Read the model definition and answer for the solid it produces. Units are mm, in the model's axes. A direction names the side the tool comes from. Coordinates: 2 decimals unless noted, no trailing zeros. Loops run counter-clockwise (first coordinate to the right, second up) from the corner with the lowest first, then second, coordinate; pieces in that order, holes last. Notation, with made-up numbers: (-23.5, -30) -> (29.5, -30) arc R24 ccw to (29.5, -2) -> close; hole circle Ø2 at (-25.75, 7). An arc over 180 degrees is marked (long way). Answer as CSV lines item,"result".
```python
from build123d import *

# Parameters (mm, degrees)
CROQUIS1_W                 = 19.8
CROQUIS1_H                 = 11.5
SALIENTE_EXTRUIR1_DEPTH    = 70.5
VACIADO1_T                 = -2
CROQUIS4_W                 = 15.8
CROQUIS4_H                 = 28
CORTAR_EXTRUIR1_DEPTH      = 2
REDONDEO1_R                = 8
CROQUIS5_W                 = 15.8
CROQUIS5_H                 = 2
SALIENTE_EXTRUIR2_DEPTH    = 2
CROQUIS6_W                 = 19.8
CROQUIS6_H                 = 10
SALIENTE_EXTRUIR4_DEPTH    = 16
SALIENTE_EXTRUIR5_DEPTH    = 19.8
CROQUIS10_R                = 3.1
CORTAR_EXTRUIR4_DEPTH      = 19.8
REDONDEO3_R                = 2
CORTAR_EXTRUIR5_DEPTH      = 52.393798264
CORTAR_EXTRUIR5_DEPTH_BACK = 52.393798264
CROQUIS11_R                = 1


with BuildPart() as part:
    # Croquis1 → Saliente-Extruir1 (new body)
    with BuildSketch(Plane(origin=(0, 0, 0), x_dir=(0, 1, 0), z_dir=(0, 0, 1))):
        Rectangle(CROQUIS1_W, CROQUIS1_H)
    extrude(amount=SALIENTE_EXTRUIR1_DEPTH)

    # Vaciado1
    vaciado1_openings = [part.faces().sort_by_distance(p)[0] for p in [
        (0, 0, 70.5),
    ]]
    offset(amount=VACIADO1_T, openings=vaciado1_openings, kind=Kind.INTERSECTION)

    # Croquis4 → Cortar-Extruir1 (cut)
    with BuildSketch(Plane.YZ.offset(5.75)):
        with Locations((0, 56.5)):
            Rectangle(CROQUIS4_W, CROQUIS4_H)
    extrude(amount=-CORTAR_EXTRUIR1_DEPTH, mode=Mode.SUBTRACT)

    # Redondeo1
    # the kernel refuses this fillet: 8 mm, written as the material it adds along each edge
    with BuildSketch(Plane(origin=(5.75, 7.9, 42.5), x_dir=(0, -1, 0), z_dir=(-1, 0, 0)), Plane(origin=(5.75, -7.9, 42.5), x_dir=(0, 0, 1), z_dir=(-1, 0, 0))) as redondeo1_piece_1:
        with BuildLine():
            CenterArc((REDONDEO1_R, REDONDEO1_R), REDONDEO1_R, 180, 90)
            Line((0, REDONDEO1_R), (0, 0))
            Line((0, 0), (REDONDEO1_R, 0))
        make_face()
    extrude(amount=2)

    # Croquis5 → Saliente-Extruir2 (add)
    with BuildSketch(Plane.YZ.offset(5.75)):
        with Locations((0, 69.5)):
            Rectangle(CROQUIS5_W, CROQUIS5_H)
    extrude(amount=-SALIENTE_EXTRUIR2_DEPTH)

    # Croquis6 → Saliente-Extruir4 (add)
    with BuildSketch(Plane(origin=(-5.75, 0, 0), x_dir=(0, -1, 0), z_dir=(-1, 0, 0))):
        with Locations((0, 25)):
            Rectangle(CROQUIS6_W, CROQUIS6_H)
    extrude(amount=SALIENTE_EXTRUIR4_DEPTH)

    # Croquis9 → Saliente-Extruir5 (add)
    with BuildSketch(Plane.XZ.offset(9.9)):
        Polygon((-5.75, 70.5), (-13.75, 30), (-5.75, 30), align=None)
        Polygon((-5.75, 0), (-13.75, 20), (-5.75, 20), align=None)
    extrude(amount=-SALIENTE_EXTRUIR5_DEPTH)

    # Croquis10 → Cortar-Extruir4 (cut)
    with BuildSketch(Plane.XZ.offset(9.9)):
        with Locations(Location((-16.745253682, 25, 0), (0, 0, 270))):
            Circle(CROQUIS10_R)
    extrude(amount=-CORTAR_EXTRUIR4_DEPTH, mode=Mode.SUBTRACT)

    # Redondeo3
    redondeo3_edges = [part.edges().sort_by_distance(p)[0] for p in [
        (-13.75, 0, 20),
        (-13.75, 0, 30),
    ]]
    fillet(redondeo3_edges, radius=REDONDEO3_R)

    # Croquis11 → Cortar-Extruir5 (cut, two sides: drawn at the far end of the back side and taken through both)
    with BuildSketch(Plane(origin=(0, 0, 25), x_dir=(0, -1, 0), z_dir=(0, 0, 1)).offset(-CORTAR_EXTRUIR5_DEPTH_BACK)):
        with Locations(Location((-5, -16.745253682, 0), (0, 0, 90))):
            Circle(CROQUIS11_R)
        with Locations(Location((5, -16.745253682, 0), (0, 0, 90))):
            Circle(CROQUIS11_R)
    extrude(amount=CORTAR_EXTRUIR5_DEPTH + CORTAR_EXTRUIR5_DEPTH_BACK, mode=Mode.SUBTRACT)


solid = part.part
```
Q1. A cutting plane is placed at D-D, the plane y = 5. Write down the section's boundary in (x, z), and give its area (3 significant figures).
Results:
outline,"(-21.75, 20) -> (-17.75, 20) -> (-17.75, 22.07) arc R3.1 cw to (-17.75, 27.93) -> (-17.75, 30) -> (-21.75, 30) -> close; (-15.75, 20) -> (-15.1, 20) arc R2 cw to (-13.25, 18.74) -> (-5.75, 0) -> (5.75, 0) -> (5.75, 44.34) -> (3.75, 44.34) -> (3.75, 2) -> (-3.75, 2) -> (-3.75, 70.5) -> (-5.75, 70.5) -> (-13.43, 31.61) arc R2 cw to (-15.39, 30) -> (-15.75, 30) -> (-15.75, 27.93) arc R3.1 cw to (-15.75, 22.07) -> close; (3.75, 68.5) -> (5.75, 68.5) -> (5.75, 70.5) -> (3.75, 70.5) -> close"
area,"614 mm²"
Q2. For a pull along Y with two mould halves and no side action, classify faces 1 (the face through (0, 7.9, 36)), 2 (the face through (-9.537, -0.139, 51.328)), 3 (the face through (-5, 9.9, 36)) as pulls with the +Y half, pulls with the -Y half, needs draft (parallel to the pull), parting line crosses it, or undercut.
Results:
face 1,"undercut"
face 2,"needs draft"
face 3,"pulls with the +Y half"
Q3. A cutting plane is placed at B-B, the plane y = 1.5. Write down the section's boundary in (x, z).
Results:
outline,"(-21.75, 20) -> (-15.1, 20) arc R2 cw to (-13.25, 18.74) -> (-5.75, 0) -> (5.75, 0) -> (5.75, 42.66) -> (3.75, 42.66) -> (3.75, 2) -> (-3.75, 2) -> (-3.75, 70.5) -> (-5.75, 70.5) -> (-13.43, 31.61) arc R2 cw to (-15.39, 30) -> (-21.75, 30) -> close; (3.75, 68.5) -> (5.75, 68.5) -> (5.75, 70.5) -> (3.75, 70.5) -> close; hole circle Ø6.2 at (-16.75, 25)"
Q4. A cutting plane is placed at C-C, the plane z = 25. Write down the section's boundary in (x, y).
Results:
outline,"(-21.75, -9.9) -> (-19.85, -9.9) -> (-19.85, 9.9) -> (-21.75, 9.9) -> close; (-13.65, -9.9) -> (5.75, -9.9) -> (5.75, 9.9) -> (-13.65, 9.9) -> close; hole (-3.75, -7.9) -> (3.75, -7.9) -> (3.75, 7.9) -> (-3.75, 7.9) -> close"
Q5. For faces 4 (the face through (4.76, 5.65, 44.94)), 5 (the face through (3.75, 0, 21)), 6 (the face through (-19, 0, 30)), determine the directions among +Z, -Z, +X, -X, +Y, -Y from which every point of the face is accessible in a straight line to the end or side of a thin tool.
Results:
face 4,"+X"
face 5,"+Z"
face 6,"+Z, -X, +Y, -Y"
Q6. A cutting plane is placed at A-A, the plane z = 16.5. Write down the section's boundary in (x, y).
Results:
outline,"(-12.35, -9.9) -> (5.75, -9.9) -> (5.75, 9.9) -> (-12.35, 9.9) -> close; hole (-3.75, -7.9) -> (3.75, -7.9) -> (3.75, 7.9) -> (-3.75, 7.9) -> close"
Q7. Find the intervals of material crossed by probe 1 along X at (y, z) = (5, 21.25); probe 2 along X at (y, z) = (-3, 25); probe 3 along Y at (x, z) = (2, 50), in increasing order. Write a range as [from, to].
Results:
probe 1,"x = [-21.75, -17.75], [-15.75, -3.75], [3.75, 5.75]"
probe 2,"x = [-21.75, -19.85], [-13.65, -3.75], [3.75, 5.75]"
probe 3,"y = [-9.9, -7.9], [7.9, 9.9]"
Q8. Given pin 1 Ø10 at (x, y) = (-10.5, -0.5) entering from +Z; pin 2 Ø3.5 at (x, y) = (-17, -0.5) entering from -Z; pin 3 Ø5 at (x, y) = (-18.5, 0.5) entering from +Z; pin 4 Ø1.6 at (y, z) = (-3, 69) entering from -X, each flat-ended and moving along its own axis, determine where each tip first touches the part or whether it passes through.
Results:
pin 1,"stops at z = 70.5"
pin 2,"stops at z = 20"
pin 3,"stops at z = 30"
pin 4,"stops at x = -6.2"
